```python
from build123d import *

# Parameters (mm, degrees)
SKETCH1_R                   = 6.477
BOSS_EXTRUDE1_DEPTH         = 9.525
FILLET1_R                   = 0.635
F_1_4_20_TAPPED_HOLE1_D     = 6.223
F_1_4_20_TAPPED_HOLE1_DEPTH = 9.525
F_1_4_20_TAPPED_HOLE1_TIP   = 1.869577816
CHAMFER1_SIZE               = 0.508


with BuildPart() as part:
    # Sketch1 → Boss-Extrude1 (new body)
    with BuildSketch(Plane(origin=(0, 0, 0), x_dir=(1, 0, 0), z_dir=(0, 1, 0))):
        Circle(SKETCH1_R)
    extrude(amount=BOSS_EXTRUDE1_DEPTH)

    # Fillet1
    fillet1_edges = [part.edges().sort_by_distance(p)[0] for p in [
        (-6.477, 9.525, 0),
    ]]
    fillet(fillet1_edges, radius=FILLET1_R)

    # 1/4-20 Tapped Hole1
    with Locations(Plane(origin=(0, 9.525, 0), x_dir=(1, 0, 0), z_dir=(0, 1, 0))):
        with Locations((0, 0)):
            Hole(F_1_4_20_TAPPED_HOLE1_D / 2, depth=F_1_4_20_TAPPED_HOLE1_DEPTH)
            with Locations((0, 0, -(F_1_4_20_TAPPED_HOLE1_DEPTH + F_1_4_20_TAPPED_HOLE1_TIP / 2))):  # 118° drill point
                Cone(0, F_1_4_20_TAPPED_HOLE1_D / 2, F_1_4_20_TAPPED_HOLE1_TIP, mode=Mode.SUBTRACT)

    # Chamfer1
    chamfer1_edges = [part.edges().sort_by_distance(p)[0] for p in [
        (3.1115, 9.525, 0),
    ]]
    chamfer(chamfer1_edges, length=CHAMFER1_SIZE)


solid = part.part
```
Here's how the part is built. I have some questions about the finished solid (model axes, mm). Give positions to 0.01 mm unless a question says otherwise; leave off trailing zeros. Write each loop counter-clockwise with the first axis right and the second up, starting at its lowest first coordinate (ties: lowest second). Pieces come first, ordered by that corner, then holes.
(1) Imagine slicing it at B-B, the plane x = 0. Write out the boundary of the cut face in (y, z) (1 decimal).
Output values:
outline: (0, -6.5) - (8.9, -6.5) arc R0.6 ccw to (9.5, -5.8) - (9.5, -3.6) - (9, -3.1) - (0, -3.1) - close; (0, 3.1) - (9, 3.1) - (9.5, 3.6) - (9.5, 5.8) arc R0.6 ccw to (8.9, 6.5) - (0, 6.5) - close
(2) Will these pins go through, and if not, where does the flat tip stop? pin 1 (4 mm diameter, centred on x = -4.5, y = 7, fed in from -Z); pin 2 (3 mm diameter, centred on x = 3, y = 4, fed in from +Z).
Output values:
pin 1: stops at z = -5.98
pin 2: stops at z = 6.3
(3) If I drill on L1, parallel to X at y = 6, z = 0; L2, parallel to X at y = 0.75, z = 2.75, over which ranges is the centre line in solid material (lowest first)?
Output values:
L1: x = -6.48 to -3.11, 3.11 to 6.48
L2: x = -5.86 to -1.46, 1.46 to 5.86
(4) Imagine slicing it at A-A, the plane z = 0. Write out the boundary of the cut face in (x, y) (1 decimal), and give its area (3 significant figures).
Output values:
outline: (-6.5, 0) - (-3.1, 0) - (-3.1, 9) - (-3.6, 9.5) - (-5.8, 9.5) arc R0.6 ccw to (-6.5, 8.9) - close; (3.1, 0) - (6.5, 0) - (6.5, 8.9) arc R0.6 ccw to (5.8, 9.5) - (3.6, 9.5) - (3.1, 9) - close
area: 63.7 mm2
(5) Imagine slicing it at C-C, the plane y = 3.5. Write out the boundary of the cut face in (x, z).
Output values:
outline: circle Ø12.95 at (0, 0); hole circle Ø6.22 at (0, 0)
(6) Thinking about a two-plate mould opening in X: for faces 1 (the face through (-1.404, 4.383, 6.323)), 2 (the face through (-3, 9.525, 3)), 3 (the face through (0.67, 4.45, 3.04)), which applies, pulls with the +X half, pulls with the -X half, needs draft (parallel to the pull), parting line crosses it, or undercut?
Output values:
face 1: parting line crosses it
face 2: needs draft
face 3: undercut
